from build123d import *

# Parameters (mm, degrees)
EXTRUDE_1_DEPTH     = 5
FILLET_1_R          = 10
CUT_EXTRUDE_1_DEPTH = 10


with BuildPart() as part:
    # 스케치1 → 보스-돌출1 (new body)
    with BuildSketch(Plane(origin=(0, 0, 0), x_dir=(0, 0, -1), z_dir=(1, 0, 0))):
        Polygon((0, 0), (-13.279056191, 23), (-13.279056191, 25), (43.279056191, 25), (43.279056191, 23), (30, 0), align=None)
    extrude(amount=EXTRUDE_1_DEPTH)

    # 필렛1
    # the kernel refuses this fillet: 10 mm, written as the material it takes off along each edge
    with BuildSketch(Plane(origin=(-6.56712034, 23, -43.279056191), x_dir=(0, 1, 0), z_dir=(1, 0, 0))) as fillet_1_piece_1:
        with BuildLine():
            CenterArc((2.725082782, 9.973678106), FILLET_1_R, 240, 25.841932763)
            Line((-2.274917218, 1.313424068), (-2.374917218, 1.140218987))
            Line((-2.374917218, 1.140218987), (-0.1, -0.173205081))
            Line((-0.1, -0.173205081), (0, -0.2))
            ThreePointArc((0, -0.2), (1, -0.2), (1.985498344, -0.199473562))
            Line((1.985498344, -0.199473562), (2, 0))
        make_face()
    extrude(amount=18.13424068, mode=Mode.SUBTRACT)
    with BuildSketch(Plane(origin=(-14.43375673, 0, -30), x_dir=(0, 0.8660254037844399, -0.499999999999998), z_dir=(1, 0, 0))) as fillet_1_piece_2:
        with BuildLine():
            CenterArc((FILLET_1_R * 0.57735026919, FILLET_1_R), FILLET_1_R, 210, 60)
            Line((-FILLET_1_R * 0.288675134595, FILLET_1_R * 0.5), (-FILLET_1_R * 0.305995642671, FILLET_1_R * 0.49))
            Line((-FILLET_1_R * 0.305995642671, FILLET_1_R * 0.49), (-FILLET_1_R * 0.0115470053838, -FILLET_1_R * 0.02))
            Line((-FILLET_1_R * 0.0115470053838, -FILLET_1_R * 0.02), (FILLET_1_R * 0.57735026919, -FILLET_1_R * 0.02))
            Line((FILLET_1_R * 0.57735026919, -FILLET_1_R * 0.02), (FILLET_1_R * 0.57735026919, 0))
        make_face()
    extrude(amount=33.867513459, mode=Mode.SUBTRACT)
    with BuildSketch(Plane(origin=(-14.43375673, 0, 0), x_dir=(0, 0.8660254037844397, 0.49999999999999833), z_dir=(1, 0, 0))) as fillet_1_piece_3:
        with BuildLine():
            CenterArc((FILLET_1_R * 0.57735026919, -FILLET_1_R), FILLET_1_R, 90, 60)
            Line((-FILLET_1_R * 0.288675134595, -FILLET_1_R * 0.5), (-FILLET_1_R * 0.305995642671, -FILLET_1_R * 0.49))
            Line((-FILLET_1_R * 0.305995642671, -FILLET_1_R * 0.49), (-FILLET_1_R * 0.0115470053838, FILLET_1_R * 0.02))
            Line((-FILLET_1_R * 0.0115470053838, FILLET_1_R * 0.02), (FILLET_1_R * 0.57735026919, FILLET_1_R * 0.02))
            Line((FILLET_1_R * 0.57735026919, FILLET_1_R * 0.02), (FILLET_1_R * 0.57735026919, 0))
        make_face()
    extrude(amount=33.867513459, mode=Mode.SUBTRACT)
    with BuildSketch(Plane(origin=(-6.56712034, 23, 13.279056191), x_dir=(0, -0.8660254037844397, -0.4999999999999979), z_dir=(1, 0, 0))) as fillet_1_piece_4:
        with BuildLine():
            CenterArc((2.626848136, 10), FILLET_1_R, 244.158067237, 25.841932763)
            Line((-1.732050808, 1), (-1.819228786, 0.82))
            ThreePointArc((-1.819228786, 0.82), (-0.966025404, 0.326794919), (-0.1, -0.173205081))
            Line((-0.1, -0.173205081), (0, -0.2))
            Line((0, -0.2), (2.626848136, -0.2))
            Line((2.626848136, -0.2), (2.626848136, 0))
        make_face()
    extrude(amount=18.13424068, mode=Mode.SUBTRACT)

    # 스케치2 → 컷-돌출1 (cut)
    with BuildSketch(Plane(origin=(5, 0, 0), x_dir=(0, 0, -1), z_dir=(1, 0, 0))):
        Polygon((19.618802154, 20), (10.381197846, 20), (5.762395693, 12), (10.381197846, 4), (19.618802154, 4), (24.237604307, 12), align=None)
    extrude(amount=-CUT_EXTRUDE_1_DEPTH, mode=Mode.SUBTRACT)


solid = part.part
Can you work these out from the model? Positions are in its coordinate system, mm. A direction names the side the tool comes from. Give positions to 0.01 mm unless a question says otherwise; leave off trailing zeros. Write each loop counter-clockwise with the first axis right and the second up, starting at its lowest first coordinate (ties: lowest second). Pieces come first, ordered by that corner, then holes. Notation, with made-up numbers: (43.25, 81.5) -> (85.25, 81.5) arc R28 cw to (85.25, 119.5) -> close; hole circle Ø5 at (67.5, 25). An arc over 180 degrees is marked (long way). Answer as a JSON object with one key per item and string values. Group by question number.
Item 1: Please list where these lines run through material, in increasing order: line 1 (Y direction, x = 2.4, z = -17.5); line 2 (Z direction, x = 3.7, y = 19.5); line 3 (Z direction, x = 0.55, y = 10.5). Write a range as [from, to].
Item 2: We'd pull the mould along Z, two halves only. Please class faces 1 (the face through (3, 20, -15)), 2 (the face through (2.465, 22.758, -42.855)), 3 (the face through (2.46, 12.75, 7.36)): +Z half, -Z half, draft (parallel to the pull), parting line (faces both ways), or undercut.
Item 3: Suppose I cut it at D-D (z = -36). Please give me the cut outline in (x, y), plus the area to 3 significant figures.
Item 4: I'm going to push a flat-ended pin straight in: P1, Ø2, axis at x = 1.5, y = 7.5, coming from the +Z side. Where does the tip first touch, or does it pass through?
Item 5: Suppose I cut it at C-C (z = -23). Please give me the cut outline in (x, y), plus the area to 3 significant figures.
Item 6: Suppose I cut it at A-A (x = 1.9). Please give me the cut outline in (y, z), plus the area to 3 significant figures.
Item 7: For faces 4 (the face through (2.46, 1.3, -29.16)), 5 (the face through (2.535, 15.944, -21.961)), which set-ups out of +Z, -Z, +X, -X, +Y, -Y let a thin tool reach every point of the face, with its end or its side?
Item 8: Suppose I cut it at B-B (y = 19). Please give me the cut outline in (x, z), plus the area to 3 significant figures.
Findings:
{
 "1": {"line 1": "y = [0, 4], [20, 25]", "line 2": "z = [-41.26, -19.91], [-10.09, 11.26]", "line 3": "z = [-36.06, -23.37], [-6.63, 6.06]"},
 "2": {"face 1": "undercut", "face 2": "-Z half", "face 3": "+Z half"},
 "3": {"outline": "(0, 10.39) -> (5, 10.39) -> (5, 25) -> (0, 25) -> close", "area": "73.0 mm²"},
 "4": {"P1": "stops at z = 4.91"},
 "5": {"outline": "(0, 0) -> (5, 0) -> (5, 9.86) -> (0, 9.86) -> close; (0, 14.14) -> (5, 14.14) -> (5, 25) -> (0, 25) -> close", "area": "104 mm²"},
 "6": {"outline": "(0, -24.23) arc R10 ccw to (5, -32.89) -> (20.73, -41.97) arc R10 ccw to (25, -43.28) -> (25, 13.28) arc R10 ccw to (20.73, 11.97) -> (5, 2.89) arc R10 ccw to (0, -5.77) -> close; hole (4, -19.62) -> (12, -24.24) -> (20, -19.62) -> (20, -10.38) -> (12, -5.76) -> (4, -10.38) -> close", "area": "875 mm²"},
 "7": {"face 4": "-Z, +X, -X, -Y", "face 5": "+X, -X"},
 "8": {"outline": "(0, -40.97) -> (5, -40.97) -> (5, -20.2) -> (0, -20.2) -> close; (0, -9.8) -> (5, -9.8) -> (5, 10.97) -> (0, 10.97) -> close", "area": "208 mm²"}
}
